The model under review builds one solid part; all positions refer to its coordinate system, in mm. Coordinates: 2 decimals unless noted, no trailing zeros. Loops run counter-clockwise (first coordinate to the right, second up) from the corner with the lowest first, then second, coordinate; pieces in that order, holes last. Notation, with made-up numbers: M -35,27.5 L 15,27.5 A28 cw 15,66.5 Z; hole C 71.25,27.5 d3. An arc over 180 degrees is marked long. Return JSON: item names as keys, results as strings.
```python
from build123d import *

# Parameters (mm, degrees)
BOSS_EXTRUDE1_DEPTH = 2.54


with BuildPart() as part:
    # Sketch1 → Boss-Extrude1 (new body)
    with BuildSketch(Plane(origin=(0, 0, 0), x_dir=(0, 0, -1), z_dir=(1, 0, 0))):
        with BuildLine():
            Line((12.7, 0), (82.55, 0))
            ThreePointArc((82.55, 0), (91.530256121, 3.719743879), (95.25, 12.7))
            Line((95.25, 12.7), (95.25, 184.15))
            ThreePointArc((95.25, 184.15), (91.530256121, 193.130256121), (82.55, 196.85))
            Line((82.55, 196.85), (12.7, 196.85))
            ThreePointArc((12.7, 196.85), (3.719743879, 193.130256121), (0, 184.15))
            Line((0, 184.15), (0, 12.7))
            ThreePointArc((0, 12.7), (3.719743879, 3.719743879), (12.7, 0))
        make_face()
        with BuildLine():
            Line((82.55, 6.35), (12.7, 6.35))
            ThreePointArc((12.7, 6.35), (6.35, 12.7), (12.7, 19.05))
            Line((12.7, 19.05), (82.55, 19.05))
            ThreePointArc((82.55, 19.05), (88.9, 12.7), (82.55, 6.35))
        make_face(mode=Mode.SUBTRACT)
        with BuildLine():
            Line((82.55, 177.8), (12.7, 177.8))
            ThreePointArc((12.7, 177.8), (6.35, 184.15), (12.7, 190.5))
            Line((12.7, 190.5), (82.55, 190.5))
            ThreePointArc((82.55, 190.5), (88.9, 184.15), (82.55, 177.8))
        make_face(mode=Mode.SUBTRACT)
    extrude(amount=BOSS_EXTRUDE1_DEPTH)


solid = part.part
```
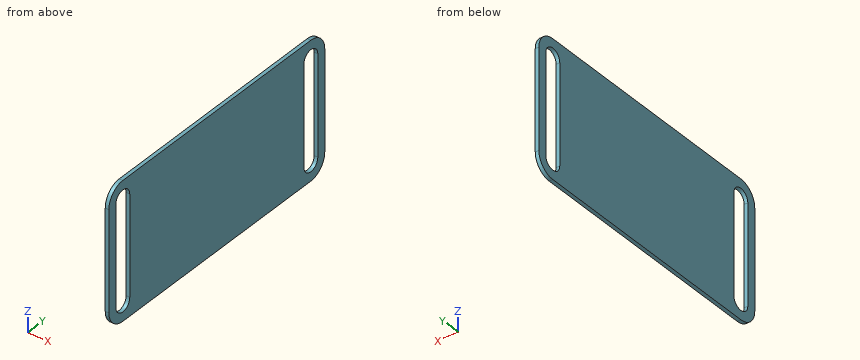
1. Add section B-B on x = 1.8. Give the boundary of the cut face in (y, z), plus the area to 3 significant figures.
Check values:
{"outline": "M 0,-82.55 A12.7 ccw 12.7,-95.25 L 184.15,-95.25 A12.7 ccw 196.85,-82.55 L 196.85,-12.7 A12.7 ccw 184.15,0 L 12.7,0 A12.7 ccw 0,-12.7 Z; hole M 6.35,-82.55 A6.35 ccw 19.05,-82.55 L 19.05,-12.7 A6.35 ccw 6.35,-12.7 Z; hole M 177.8,-82.55 A6.35 ccw 190.5,-82.55 L 190.5,-12.7 A6.35 ccw 177.8,-12.7 Z", "area": "16,600 mm²"}
2. To check wall thickness, follow line 1 (Y direction, x = 0.8, z = -14); line 2 (Y direction, x = 2, z = -91). State the ranges of each line that lie inside material, in increasing order.
Check values:
{"line 1": "0 to 6.35, 19.05 to 177.8, 190.5 to 196.85", "line 2": "3.22 to 193.63"}
3. Add section C-C on z = -87. Give the boundary of the cut face in (x, y).
Check values:
{"outline": "M 0,0.81 L 2.54,0.81 L 2.54,8.17 L 0,8.17 Z; M 0,17.23 L 2.54,17.23 L 2.54,179.62 L 0,179.62 Z; M 0,188.68 L 2.54,188.68 L 2.54,196.04 L 0,196.04 Z"}
4. Add section A-A on z = -18.5. Give the boundary of the cut face in (x, y).
Check values:
{"outline": "M 0,0 L 2.54,0 L 2.54,6.35 L 0,6.35 Z; M 0,19.05 L 2.54,19.05 L 2.54,177.8 L 0,177.8 Z; M 0,190.5 L 2.54,190.5 L 2.54,196.85 L 0,196.85 Z"}
